CAD build for the part. Positions are in the model's coordinates, mm. Coordinates: 2 decimals unless noted, no trailing zeros. Loops run counter-clockwise (first coordinate to the right, second up) from the corner with the lowest first, then second, coordinate; pieces in that order, holes last. Notation, with made-up numbers: (-27, 63.5) -> (27, 63.5) arc R30 cw to (27, 97.5) -> close; hole circle Ø5 at (-8.75, 79). An arc over 180 degrees is marked (long way). Return JSON: item names as keys, results as strings. Group by question number.
(1) Flat gauge pins, fed straight in: pin 1 Ø1.5 at (x, z) = (-6.5, 2) entering from -Y; pin 2 Ø1.5 at (x, z) = (-1, 2) entering from +Y. Where does each tip first touch, or does it go through?
(2) Probe L1, parallel to Y at x = -11, z = 2.5; L2, parallel to Y at x = -1.5, z = 0.4; L3, parallel to X at y = 23.5, z = 2.45. List the from-to ranges inside material, lowest first.
(3) Saw through at D-D on y = 3. Write the cut outline in (x, z).
(4) Saw through at B-B on y = 8. Write the cut outline in (x, z).
(5) Saw through at A-A on z = 1.65. Write the cut outline in (x, y).
(6) Saw through at C-C on x = -17. Write the cut outline in (y, z), then the cut area to 3 significant figures.
```python
from build123d import *

# Parameters (mm, degrees)
EXTRUDE_1_DEPTH     = 3
CUT_EXTRUDE_1_DEPTH = 56.259583795


with BuildPart() as part:
    # 草图1 → 凸台-拉伸1 (new body)
    with BuildSketch(Plane.XY):
        with BuildLine():
            ThreePointArc((-35.539590168, 31.129951211), (-39.558828054, 16.129951211), (-35.539590168, 1.129951211))
            ThreePointArc((-35.539590168, 1.129951211), (-5.539590168, -6.207235816), (24.460409832, 1.129951211))
            ThreePointArc((24.460409832, 1.129951211), (28.479647718, 16.129951211), (24.460409832, 31.129951211))
            ThreePointArc((24.460409832, 31.129951211), (-5.539590168, 38.467138237), (-35.539590168, 31.129951211))
        make_face()
    extrude(amount=EXTRUDE_1_DEPTH)

    # 草图2 → 切除-拉伸1 (cut, through all)
    with BuildSketch(Plane.XY.offset(3)):
        with BuildLine():
            Line((-15.539590168, 26.129951211), (4.460409832, 26.129951211))
            ThreePointArc((4.460409832, 26.129951211), (14.460409832, 16.129951211), (4.460409832, 6.129951211))
            Line((4.460409832, 6.129951211), (-15.539590168, 6.129951211))
            ThreePointArc((-15.539590168, 6.129951211), (-25.539590168, 16.129951211), (-15.539590168, 26.129951211))
        make_face()
    extrude(amount=-CUT_EXTRUDE_1_DEPTH, mode=Mode.SUBTRACT)


solid = part.part
```
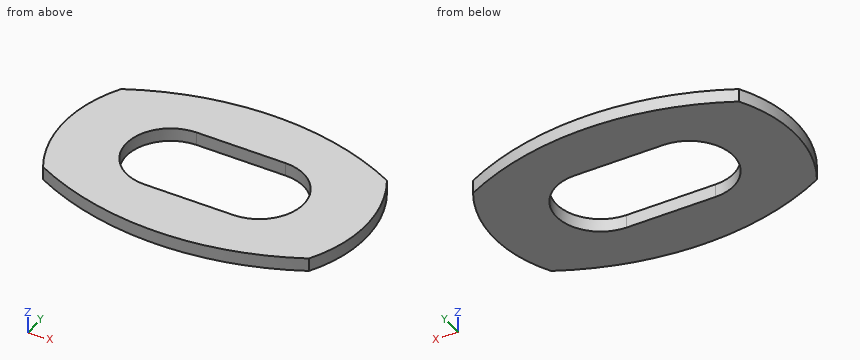
Geometry results:
{
 "1": {"pin 1": "y = -6.21", "pin 2": "y = 38.36"},
 "2": {"L1": "-5.98 to 6.13, 26.13 to 38.24", "L2": "-6.08 to 6.13, 26.13 to 38.34", "L3": "-38.64 to -22.3, 11.22 to 27.56"},
 "3": {"outline": "(-36.53, 0) -> (25.45, 0) -> (25.45, 3) -> (-36.53, 3) -> close"},
 "4": {"outline": "(-38.44, 0) -> (-21.36, 0) -> (-21.36, 3) -> (-38.44, 3) -> close; (10.28, 0) -> (27.36, 0) -> (27.36, 3) -> (10.28, 3) -> close"},
 "5": {"outline": "(-35.54, 1.13) arc R65 ccw to (24.46, 1.13) arc R30 ccw to (24.46, 31.13) arc R65 ccw to (-35.54, 31.13) arc R30 ccw to start; hole (-15.54, 6.13) -> (4.46, 6.13) arc R10 ccw to (4.46, 26.13) -> (-15.54, 26.13) arc R10 ccw to start"},
 "6": {"outline": "(-5.19, 0) -> (6.24, 0) -> (6.24, 3) -> (-5.19, 3) -> close; (26.02, 0) -> (37.45, 0) -> (37.45, 3) -> (26.02, 3) -> close", "area": "68.6 mm²"}
}
